Autodesk Inventor part; units mm, degrees
ref_plane "YZ Plane" through (0, 0, 0) normal (1, 0, 0) x (0, 1, 0)
ref_plane "XZ Plane" through (0, 0, 0) normal (0, 1, 0) x (-1, 0, 0)
ref_plane "XY Plane" through (0, 0, 0) normal (0, 0, 1) x (1, 0, 0)
sketch "Sketch1" plane through (0, 0, 0) normal (0, 0, 1) x (1, 0, 0)
  line L0 (0, 519.43) -> (0, -494.03)
  line L1 (-334.6907, 0) -> (334.6907, 0)
  line L2 (239.0648, -349.25) -> (-239.0648, -349.25)
  line L3 (-239.0648, -349.25) -> (-239.0648, 349.25)
  line L4 (-239.0648, 349.25) -> (239.0648, 349.25)
  line L5 (239.0648, 349.25) -> (239.0648, -349.25)
  line L6 (239.0648, -349.25) -> (-239.0648, 349.25) construction
  line L7 (-239.0648, -349.25) -> (239.0648, 349.25) construction
  line L8 (220.345, -330.5302) -> (-220.345, -330.5302) construction
  line L9 (-220.345, -330.5302) -> (-220.345, 330.5302) construction
  line L10 (-220.345, 330.5302) -> (220.345, 330.5302) construction
  line L11 (220.345, 330.5302) -> (220.345, -330.5302) construction
  line L12 (220.345, -330.5302) -> (-220.345, 330.5302) construction
  line L13 (-220.345, -330.5302) -> (220.345, 330.5302) construction
  line L14 (47.625, 374.65) -> (-47.625, 374.65)
  line L15 (-47.625, 374.65) -> (-47.625, 349.25)
  line L16 (-47.625, 349.25) -> (47.625, 349.25)
  line L17 (47.625, 349.25) -> (47.625, 374.65)
  line L18 (47.625, 374.65) -> (-47.625, 349.25) construction
  line L19 (-47.625, 374.65) -> (47.625, 349.25) construction
  point P0 (0, 0)
  point P1 (-156.5148, 330.5302)
  point P2 (0, 330.5302)
  point P3 (156.5148, 330.5302)
  point P4 (-156.5148, -330.5302)
  point P5 (0, -330.5302)
  point P6 (156.5148, -330.5302)
  point P7 (-220.345, 143.51)
  point P8 (-220.345, -143.51)
  point P9 (220.345, 143.51)
  point P10 (220.345, -117.0967)
  point P11 (-220.345, 0)
  point P12 (0, 361.95)
  point P13 (0, 361.6198)
  dimension "d0" = 478.1296
  dimension "d1" = 698.5
  dimension "d3" = 18.7198
  dimension "d4" = 18.7198
  dimension "d7" = 143.51
  dimension "d8" = 143.51
  dimension "d10" = 205.74
  dimension "d20" = 82.55
  dimension "d21" = 82.55
  dimension "d23" = 95.25
  dimension "d24" = 25.4
  dimension "d27" = 12.3698
extrude "Extrusion1" add sketch "Sketch1" against normal blind 3.175
hole "Hole1" at (-156.5148, -330.5302, 0) at (156.5148, -330.5302, 0) at (220.345, 143.51, 0) at (220.345, -117.0967, 0) at (-220.345, 143.51, 0) at (-220.345, -143.51, 0) at (-220.345, 330.5302, 0) at (220.345, 330.5302, 0) at (0, 361.6198, 0) direction (0, 0, -1) diameter 8.255 end through all
fillet "Fillet1" radius 9.525 4 edges at (-239.0648, 349.25, -1.5875) (239.0648, 349.25, -1.5875) (239.0648, -349.25, -1.5875) (-239.0648, -349.25, -1.5875)
fillet "Fillet2" radius 3.175 4 edges at (47.625, 374.65, -1.5875) (47.625, 349.25, -1.5875) (-47.625, 374.65, -1.5875) (-47.625, 349.25, -1.5875)
properties material "ALUMINUM, 6061-T651"
CAD build for the part. Positions are in the model's coordinates, mm. Round coordinates to 2 decimals unless told otherwise and drop trailing zeros. Loops run counter-clockwise (first coordinate to the right, second up) from the corner with the lowest first, then second, coordinate; pieces in that order, holes last. Notation, with made-up numbers: M 39,-11 L 84,-11 A30 ccw 84,23 Z; hole C -32.5,-21.5 d2. An arc over 180 degrees is marked long. Use a Markdown table: item, result. Add a question column.
(1) Drill centre lines: line 1 (X direction, y = 143.51, z = -2.1); line 2 (X direction, y = -144.5, z = -1.8); line 3 (X direction, y = 147, z = -1.85). Where is each one in solid material? Low to high.
(2) Cut at B-B (x = -199). Give the cut face in (y, z) (3 decimals), and give its area (3 significant figures).
(3) Flat gauge pins, fed straight in: pin 1 (1 mm diameter, centred on x = 98.5, z = -2.5, fed in from +Y); pin 2 (7.5 mm diameter, centred on x = 156.51, y = -330.53, fed in from -Z). Where does each tip first touch, or does it go through?
(4) Cut at A-A (z = -0.7). State how many separate pieces and enclosed holes the cut face has, and give its area (3 significant figures).
Geometry says:
| question | item | result |
|---|---|---|
| 1 | line 1 | x = -239.06 to -224.47, -216.22 to 216.22, 224.47 to 239.06 |
| 1 | line 2 | x = -239.06 to -224.35, -216.34 to 239.06 |
| 1 | line 3 | x = -239.06 to -222.55, -218.14 to 218.14, 222.55 to 239.06 |
| 2 | outline | M -349.25,-3.175 L 349.25,-3.175 L 349.25,0 L -349.25,0 Z |
| 2 | area | 2,220 mm² |
| 3 | pin 1 | stops at y = 349.25 |
| 3 | pin 2 | passes through |
| 4 | separate pieces | 1 |
| 4 | enclosed holes | 9 |
| 4 | area | 336,000 mm² |
